Model file for the job. Use its own axes, mm. Face numbers are marked on the shaded views. A direction names the side the tool comes from. Round coordinates to 2 decimals unless told otherwise and drop trailing zeros. Loops run counter-clockwise (first coordinate to the right, second up) from the corner with the lowest first, then second, coordinate; pieces in that order, holes last. Notation, with made-up numbers: M 48.5,59 L 59.5,59 A33 cw 59.5,92 Z; hole C 45.25,55.25 d1. An arc over 180 degrees is marked long. Use a Markdown table: item, result. Add a question column.
Item 1: Saw through at B-B on z = -19. Write the cut outline in (x, y).
Item 2: Saw through at A-A on x = 24. Write the cut outline in (y, z), then the cut area to 3 significant figures.
Item 3: Wall check: L1, parallel to Y at x = 7, z = -2.4 (3 decimals); L2, parallel to Z at x = 30, y = 6; L3, parallel to Y at x = 30, z = -15. Give the ranges that are in metal, low to high. Write a range as from..to.
Item 4: Pin check, flat tips, straight feed: P1, Ø4.5, axis at x = 53, y = 6.5, coming from the -Z side; P2, Ø5, axis at y = 9, z = -10, coming from the -X side; P3, Ø1, axis at x = 4, z = -15.5, coming from the +Y side. Stop position of each tip, or through.
Item 5: Saw through at C-C on z = -9. Write the cut outline in (x, y).
Item 6: Tool access for the marked faces 1 and 2: list every direction of +Z, -Z, +X, -X, +Y, -Y with a clear straight run to the whole face (end or side of a thin tool).
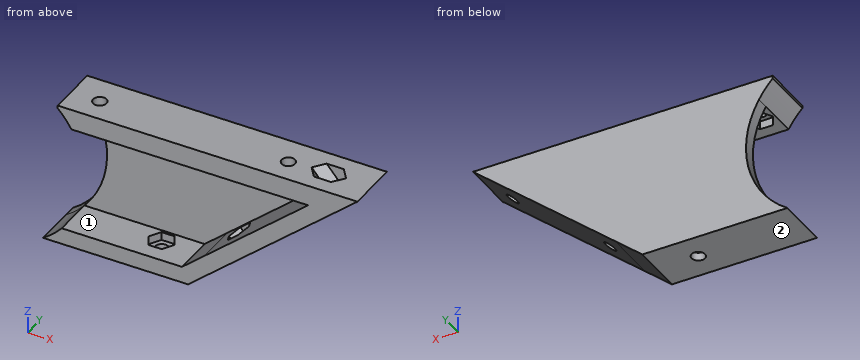
```python
from build123d import *

# Parameters (mm, degrees)
SALIENTE_EXTRUIR1_DEPTH = 12.75
CORTAR_EXTRUIR1_REACH   = 31.62
CROQUIS2_R              = 1.625
CROQUIS3_R              = 22.5
CORTAR_EXTRUIR2_DEPTH   = 13.75
SALIENTE_EXTRUIR2_DEPTH = 3
SALIENTE_EXTRUIR3_DEPTH = 9.75
CROQUIS6_R              = 1.625
CORTAR_EXTRUIR3_DEPTH   = 10
CORTAR_EXTRUIR4_START   = -2
CORTAR_EXTRUIR4_DEPTH   = 10
CORTAR_EXTRUIR5_START   = -2
CORTAR_EXTRUIR5_DEPTH   = 10
CORTAR_EXTRUIR6_DEPTH   = 2
CORTAR_EXTRUIR7_REACH   = 37.25
CROQUIS10_R             = 1.625
CORTAR_EXTRUIR8_DEPTH   = 2


with BuildPart() as part:
    # Croquis1 → Saliente-Extruir1 (new body)
    with BuildSketch(Plane(origin=(0, 0, 0), x_dir=(1, 0, 0), z_dir=(0, 1, 0))):
        Polygon((0, 0), (72.78319995, 0), (38.224450787, 29.62043043), (35.621353918, 26.5833452), (60.803074847, 5), (0, 5), align=None)
    extrude(amount=SALIENTE_EXTRUIR1_DEPTH)

    # Croquis2 → Cortar-Extruir1 (cut, up to next)
    with BuildSketch(Plane.XY, mode=Mode.PRIVATE) as cortar_extruir1_sk1:
        with Locations((52.78319995, 5.75)):
            Circle(CROQUIS2_R)
    cortar_extruir1_tool1 = extrude(cortar_extruir1_sk1.sketch, amount=-CORTAR_EXTRUIR1_REACH, mode=Mode.PRIVATE) & part.part
    add(cortar_extruir1_tool1.solids().sort_by_distance((52.7832, 5.75, 0))[0], mode=Mode.SUBTRACT)
    # Croquis2 → Cortar-Extruir1 (cut, up to next)
    with BuildSketch(Plane.XY, mode=Mode.PRIVATE) as cortar_extruir1_sk2:
        with Locations((6.99999995, 5.75)):
            Circle(CROQUIS2_R)
    cortar_extruir1_tool2 = extrude(cortar_extruir1_sk2.sketch, amount=-CORTAR_EXTRUIR1_REACH, mode=Mode.PRIVATE) & part.part
    add(cortar_extruir1_tool2.solids().sort_by_distance((7, 5.75, 0))[0], mode=Mode.SUBTRACT)

    # Croquis3 → Cortar-Extruir2 (cut, through all)
    with BuildSketch(Plane(origin=(0, 12.75, 0), x_dir=(1, 0, 0), z_dir=(0, 1, 0))):
        with Locations((-16, 16.5)):
            Circle(CROQUIS3_R)
    extrude(amount=-CORTAR_EXTRUIR2_DEPTH, mode=Mode.SUBTRACT)

    # Croquis4 → Saliente-Extruir2 (add)
    with BuildSketch(Plane(origin=(0, 12.75, 0), x_dir=(1, 0, 0), z_dir=(0, 1, 0))):
        with BuildLine():
            Line((38.224450787, 29.62043043), (31.656319269, 35.25))
            Line((31.656319269, 35.25), (-3.562657036, 35.25))
            ThreePointArc((-3.562657036, 35.25), (5.936291456, 21.504909307), (3.339079606, 5))
            Line((3.339079606, 5), (60.803074847, 5))
            Line((60.803074847, 5), (35.621353918, 26.5833452))
            Line((35.621353918, 26.5833452), (38.224450787, 29.62043043))
        make_face()
    extrude(amount=-SALIENTE_EXTRUIR2_DEPTH)

    # Croquis5 → Saliente-Extruir3 (add)
    with BuildSketch(Plane.XZ.offset(-9.75)):
        with BuildLine():
            Line((-3.562657036, -35.25), (31.656319269, -35.25))
            Line((31.656319269, -35.25), (38.224450787, -29.62043043))
            Line((38.224450787, -29.62043043), (35.621353918, -26.5833452))
            Line((35.621353918, -26.5833452), (30.17667434, -31.25))
            Line((30.17667434, -31.25), (0.990806338, -31.25))
            ThreePointArc((0.990806338, -31.25), (-1.15062315, -33.404023402), (-3.562657036, -35.25))
        make_face()
    extrude(amount=SALIENTE_EXTRUIR3_DEPTH)

    # Croquis6 → Cortar-Extruir3 (cut)
    with BuildSketch(Plane(origin=(30.824200619, 0, -35.963211942), x_dir=(-0.759271307, 0, -0.650774217), z_dir=(0.650774217, 0, -0.759271307))):
        with Locations((-47.262195378, 6.375)):
            Circle(CROQUIS6_R)
        with Locations((-16.095943758, 6.375)):
            Circle(CROQUIS6_R)
    extrude(amount=-CORTAR_EXTRUIR3_DEPTH, mode=Mode.SUBTRACT)

    # Croquis7 → Cortar-Extruir4 (cut)
    with BuildSketch(Plane(origin=(28.22110375, 0, -32.926126712), x_dir=(0.759271307, 0, 0.650774217), z_dir=(-0.650774217, 0, 0.759271307)).offset(CORTAR_EXTRUIR4_START)):
        Polygon((48.849908618, 3.625), (50.437621859, 6.375), (48.849908618, 9.125), (45.674482138, 9.125), (44.086768898, 6.375), (45.674482138, 3.625), align=None)
    extrude(amount=CORTAR_EXTRUIR4_DEPTH, mode=Mode.SUBTRACT)

    # Croquis8 → Cortar-Extruir5 (cut)
    with BuildSketch(Plane(origin=(28.22110375, 0, -32.926126712), x_dir=(0.759271307, 0, 0.650774217), z_dir=(-0.650774217, 0, 0.759271307)).offset(CORTAR_EXTRUIR5_START)):
        Polygon((17.683656999, 3.625), (19.271370239, 6.375), (17.683656999, 9.125), (14.508230518, 9.125), (12.920517278, 6.375), (14.508230518, 3.625), align=None)
    extrude(amount=CORTAR_EXTRUIR5_DEPTH, mode=Mode.SUBTRACT)

    # Croquis9 → Cortar-Extruir6 (cut)
    with BuildSketch(Plane(origin=(0, 0, -5), x_dir=(-1, 0, 0), z_dir=(0, 0, -1))):
        Polygon((-5.41228671, 3), (-3.824573469, 5.75), (-5.41228671, 8.5), (-8.58771319, 8.5), (-10.175426431, 5.75), (-8.58771319, 3), align=None)
        Polygon((-51.19548671, 3), (-49.607773469, 5.75), (-51.19548671, 8.5), (-54.37091319, 8.5), (-55.958626431, 5.75), (-54.37091319, 3), align=None)
    extrude(amount=-CORTAR_EXTRUIR6_DEPTH, mode=Mode.SUBTRACT)

    # Croquis10 → Cortar-Extruir7 (cut, up to next)
    with BuildSketch(Plane(origin=(0, 0, -35.25), x_dir=(-1, 0, 0), z_dir=(0, 0, -1)), mode=Mode.PRIVATE) as cortar_extruir7_sk1:
        with Locations((-21.656319269, 6.375)):
            Circle(CROQUIS10_R)
    cortar_extruir7_tool1 = extrude(cortar_extruir7_sk1.sketch, amount=-CORTAR_EXTRUIR7_REACH, mode=Mode.PRIVATE) & part.part
    add(cortar_extruir7_tool1.solids().sort_by_distance((21.656319, 6.375, -35.25))[0], mode=Mode.SUBTRACT)

    # Croquis11 → Cortar-Extruir8 (cut)
    with BuildSketch(Plane.XY.offset(-31.25)):
        Polygon((23.24403251, 3.625), (24.83174575, 6.375), (23.24403251, 9.125), (20.068606029, 9.125), (18.480892789, 6.375), (20.068606029, 3.625), align=None)
    extrude(amount=-CORTAR_EXTRUIR8_DEPTH, mode=Mode.SUBTRACT)


solid = part.part
```
Entries:
| question | item | result |
|---|---|---|
| 1 | outline | M 6.36,9.75 L 44.47,9.75 L 44.47,0 L 50.62,0 L 50.62,12.75 L 6.36,12.75 Z |
| 2 | outline | M 0,-35.25 L 12.75,-35.25 L 12.75,0 L 0,0 L 0,-5 L 9.75,-5 L 9.75,-31.25 L 7.82,-31.25 L 7.82,-33.25 L 4.93,-33.25 L 4.93,-31.25 L 0,-31.25 Z |
| 2 | area | 188 mm2 |
| 3 | L1 | 0..4.125, 7.375..12.75 |
| 3 | L2 | -35.25..-31.25, -5..0 |
| 3 | L3 | 9.75..12.75 |
| 4 | P1 | z = -18.88 |
| 4 | P2 | x = 4.67 |
| 4 | P3 | through |
| 5 | outline | M 5.21,9.75 L 56.14,9.75 L 56.14,0 L 62.28,0 L 62.28,12.75 L 5.21,12.75 Z |
| 6 | face 1 | -X, -Y |
| 6 | face 2 | -Z, +X, -X, +Y, -Y |
